Source: CAD feature listing. Evaluate the final solid. Frame: model axes, mm. A direction names the side the tool comes from. Give positions to 0.01 mm unless a question says otherwise; leave off trailing zeros. Write each loop counter-clockwise with the first axis right and the second up, starting at its lowest first coordinate (ties: lowest second). Pieces come first, ordered by that corner, then holes. Notation, with made-up numbers: M 23.5,-9 L 55.5,-9 A18 ccw 55.5,11 Z; hole C 48,46 d6. An arc over 180 degrees is marked long. Use CSV: the item, a comma, the result in double quotes. Start each with the question number.
from build123d import *

# Parameters (mm, degrees)
F0_R      = 4
F1_DEPTH  = 136
F2_R      = 15
F3_DEPTH  = 10
F4_SIZE   = 9.99999
F5_R      = 25
F5_R_2    = 15
F6_DEPTH  = 7.5
F7_R      = 2.25
F8_DEPTH  = 153.501
F9_W      = 2.5
F9_H      = 5
F10_DEPTH = 5


# Not quite as in the source:
# - a fillet or chamfer is up to 0.001 mm smaller than in the source, because OpenCascade refuses the exact size


with BuildPart() as f1:
    # F0 (on Top) → F1 (new body)
    with BuildSketch(Plane.XY):
        Circle(F0_R)
    extrude(amount=F1_DEPTH)

    # F2 (on Top) → F3 (join)
    with BuildSketch(Plane.XY):
        Circle(F2_R)
    extrude(amount=-F3_DEPTH)

    # F4 (size 10 in the source; OpenCascade refuses exactly that, so slightly less here)
    f4_edges = [f1.edges().sort_by_distance(p)[0] for p in [
        (-15, 0, 0),
    ]]
    chamfer(f4_edges, length=F4_SIZE)

    # F5 (on face) → F6 (join)
    with BuildSketch(Plane(origin=(0, 0, -10), x_dir=(1, 0, 0), z_dir=(0, 0, -1))):
        Circle(F5_R)
        Circle(F5_R_2, mode=Mode.SUBTRACT)
        Circle(F5_R_2)
    extrude(amount=F6_DEPTH)

    # F7 (on face) → F8 (cut, through all)
    with BuildSketch(Plane(origin=(0, 0, -17.5), x_dir=(1, 0, 0), z_dir=(0, 0, -1))):
        with Locations((-20, 0)):
            Circle(F7_R)
        with Locations((0, 20)):
            Circle(F7_R)
        with Locations((20, 0)):
            Circle(F7_R)
        with Locations((0, -20)):
            Circle(F7_R)
    extrude(amount=-F8_DEPTH, mode=Mode.SUBTRACT)

    # F9 (on face) → F10 (cut)
    with BuildSketch(Plane.XY):
        with Locations((0, 5.8)):
            Rectangle(F9_W, F9_H)
        Polygon((-2.2328838325, 2.7325317547), (-6.5630108514, 5.2325317547), (-7.8130108514, 3.0674682453), (-3.4828838325, 0.5674682453), align=None)
        Polygon((-3.4828838325, -0.5674682453), (-7.8130108514, -3.0674682453), (-6.5630108514, -5.2325317547), (-2.2328838325, -2.7325317547), align=None)
        with Locations((0, -5.8)):
            Rectangle(F9_W, F9_H)
        Polygon((2.2328838325, -2.7325317547), (6.5630108514, -5.2325317547), (7.8130108514, -3.0674682453), (3.4828838325, -0.5674682453), align=None)
        Polygon((3.4828838325, 0.5674682453), (7.8130108514, 3.0674682453), (6.5630108514, 5.2325317547), (2.2328838325, 2.7325317547), align=None)
    extrude(amount=-F10_DEPTH, mode=Mode.SUBTRACT)


solid = f1.part
1. Section C-C on z = 33. Return loops of the section in (x, y).
2. Section A-A on x = -20. Return loops of the section in (y, z).
3. Access query for faces 4 (the cylindrical face through (-0.488, 22.196, -13.802)), 5 (the flat face through (3.947, 3.722, -3.021)). Directions: +Z, -Z, +X, -X, +Y, -Y. A direction counts if a zero-diameter tool reaches every point of the face in a straight line with its end or side. Return the directions, or none.
4. First-contact query: pin 1 (1.5 mm diameter, centred on x = -16, y = 12.5, fed in from +Z); pin 2 (0.8 mm diameter, centred on x = 0.5, y = 7, fed in from +Z); pin 3 (5.5 mm diameter, centred on y = 5.5, z = -2, fed in from +X). Flat tips, straight axial feed; report the tip coordinate or a pass-through.
5. Pull-direction query (Y, two-part tool) for faces 1 (the flat face through (0, 0, -17.5)), 2 (the cylindrical face through (-0.867, -3.905, 67.048)), 3 (the flat face through (-1.25, -5, -3)); classes: released by +Y, released by -Y, zero draft, split by the parting line, or undercut.
6. Line query: probe 1 along Y at (x, z) = (0, -12); probe 2 along Y at (x, z) = (20, -14.25). Output: solid intervals per line, ascending.
Resolved:
1,outline,"C 0,0 d8"
2,outline,"M -15,-17.5 L -2.25,-17.5 L -2.25,-10 L -15,-10 Z; M 2.25,-17.5 L 15,-17.5 L 15,-10 L 2.25,-10 Z"
3,face 4,"+Z, -Z"
3,face 5,"none"
4,pin 1,"stops at z = -10"
4,pin 2,"stops at z = -5"
4,pin 3,"stops at x = 8.44"
5,face 1,"zero draft"
5,face 2,"split by the parting line"
5,face 3,"undercut"
6,probe 1,"y = -25 to -22.25, -17.75 to 17.75, 22.25 to 25"
6,probe 2,"y = -15 to -2.25, 2.25 to 15"
